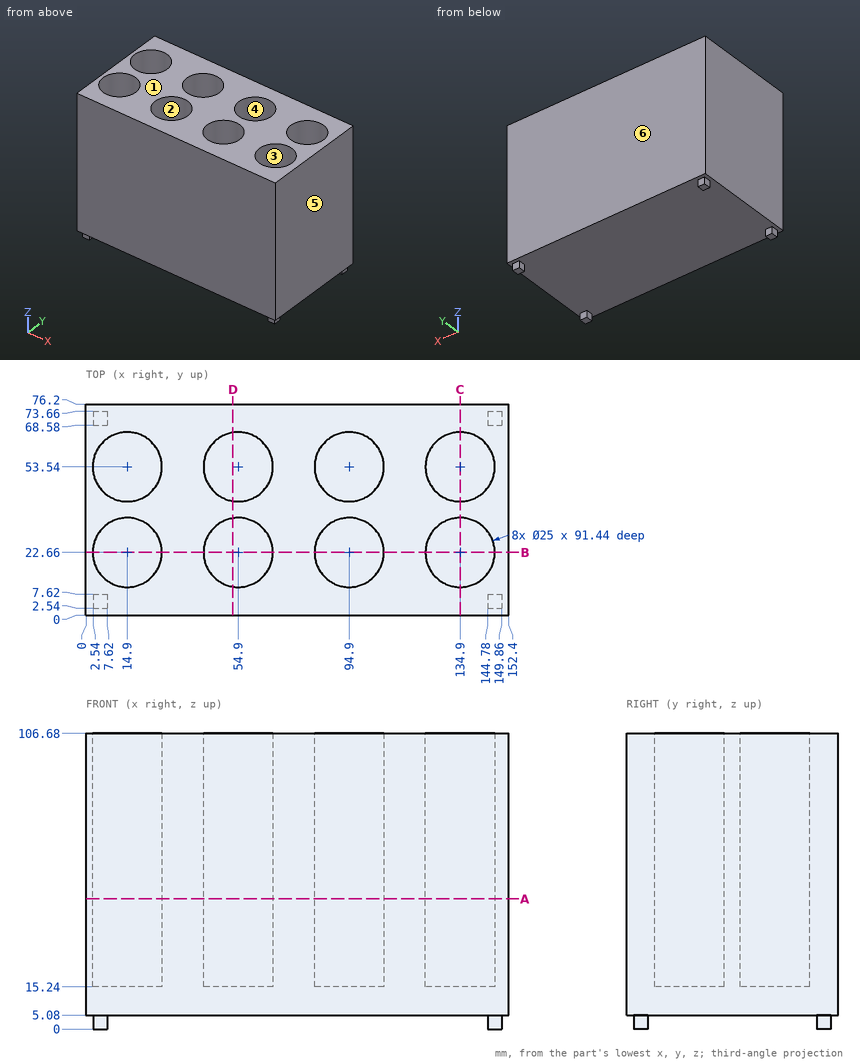
The drawing under review shows one solid part. Ordinate dimensions are in mm from its lowest x, y, z. A direction names the side the tool comes from. Round coordinates to 2 decimals unless told otherwise and drop trailing zeros. Write each loop counter-clockwise with the first axis right and the second up, starting at its lowest first coordinate (ties: lowest second). Pieces come first, ordered by that corner, then holes.
(1) Wall thickness on L1, parallel to Y at x = 134.9, z = 61.5; L2, parallel to Y at x = 54, z = 60; L3, parallel to X at y = 53, z = 50: over which ranges is each line inside the solid? List them lowest first.
(2) We need section C-C on x = 134.9. Give the boundary of the cut face in (y, z).
(3) Mouldability with a two-part tool opening along Y and no side actions: class the marked faces 3, 4, 5 and 6 as +Y half, -Y half, draft (parallel to the pull), parting line (faces both ways), or undercut.
(4) Machinability: for the marked faces 1 and 2, which of the approach directions +Z, -Z, +X, -X, +Y, -Y give a long, thin tool a straight path to every point of the face, cutting with its end or side? Answer none if there is none.
(5) We need section A-A on z = 47. Give the number of separate pieces and of enclosed holes in the cut face, and give its area (3 significant figures).
(6) Insertion check: pin 1 (23 mm diameter, centred on x = 111.5, y = 40.5, fed in from -Z); pin 2 (4 mm diameter, centred on y = 70, z = 3, fed in from -X); pin 3 (1.5 mm diameter, centred on x = 4.5, z = 2, fed in from +Y). Each pin has a flat end and moves straight along its axis. Give the tip position at first contact, or say it passes through.
(7) We need section D-D on x = 53. Give the boundary of the cut face in (y, z).
(8) We need section B-B on y = 22.66. Give the boundary of the cut face in (x, z), and give its area (3 significant figures).
Findings below:
1. L1: y = 0 to 10.16, 35.16 to 41.04, 66.04 to 76.2
1. L2: y = 0 to 10.19, 35.13 to 41.07, 66.01 to 76.2
1. L3: x = 0 to 2.41, 27.39 to 42.41, 67.39 to 82.41, 107.39 to 122.41, 147.39 to 152.4
2. outline: (0, 5.08) - (76.2, 5.08) - (76.2, 106.68) - (66.04, 106.68) - (66.04, 15.24) - (41.04, 15.24) - (41.04, 106.68) - (35.16, 106.68) - (35.16, 15.24) - (10.16, 15.24) - (10.16, 106.68) - (0, 106.68) - close
3. face 3: undercut
3. face 4: undercut
3. face 5: draft
3. face 6: +Y half
4. face 1: +Z, +X, -X, +Y, -Y
4. face 2: +Z
5. separate pieces: 1
5. enclosed holes: 8
5. area: 7,690 mm2
6. pin 1: stops at z = 5.08
6. pin 2: stops at x = 2.54
6. pin 3: stops at y = 73.66
7. outline: (0, 5.08) - (76.2, 5.08) - (76.2, 106.68) - (65.89, 106.68) - (65.89, 15.24) - (41.19, 15.24) - (41.19, 106.68) - (35.01, 106.68) - (35.01, 15.24) - (10.31, 15.24) - (10.31, 106.68) - (0, 106.68) - close
8. outline: (0, 5.08) - (152.4, 5.08) - (152.4, 106.68) - (147.4, 106.68) - (147.4, 15.24) - (122.4, 15.24) - (122.4, 106.68) - (107.4, 106.68) - (107.4, 15.24) - (82.4, 15.24) - (82.4, 106.68) - (67.4, 106.68) - (67.4, 15.24) - (42.4, 15.24) - (42.4, 106.68) - (27.4, 106.68) - (27.4, 15.24) - (2.4, 15.24) - (2.4, 106.68) - (0, 106.68) - close
8. area: 6,340 mm2
